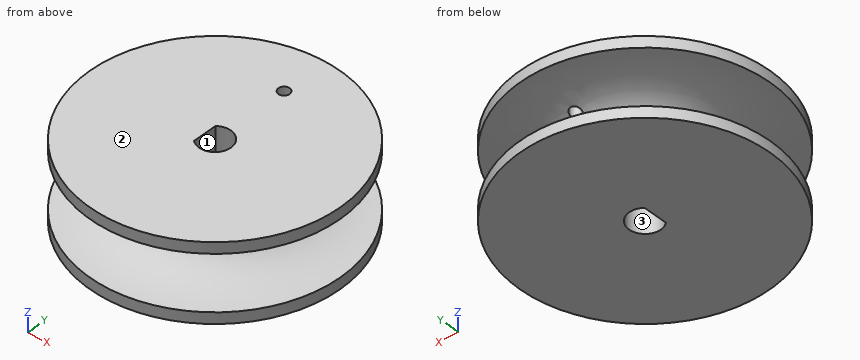
```python
from build123d import *

# Parameters (mm, degrees)
BOSS_EXTRUDE1_START = -7
BOSS_EXTRUDE1_DEPTH = 7
SKETCH8_R           = 0.5
CUT_EXTRUDE1_DEPTH  = 3


with BuildPart() as part:
    # Sketch4 → Revolve1 (revolve)
    with BuildSketch(Plane(origin=(0, 0, 0), x_dir=(0, 0, -1), z_dir=(1, 0, 0)), mode=Mode.PRIVATE) as revolve1_sk:
        with BuildLine():
            Line((-2.5, 11.25), (-3.5, 11.25))
            Line((-3.5, 11.25), (-3.5, 1.425))
            Line((-3.5, 1.425), (3.5, 1.425))
            Line((3.5, 1.425), (3.5, 11.25))
            Line((3.5, 11.25), (2.5, 11.25))
            add(Edge.make_bspline(
                [(0, 5.689829973), (2.5, 5.689829973), (2.5, 11.25)],
                knots=[0, 0, 0, 1.570796327, 1.570796327, 1.570796327], degree=2, weights=[1, 0.707106781, 1]))
            add(Edge.make_bspline(
                [(-2.5, 11.25), (-2.5, 5.689829973), (0, 5.689829973)],
                knots=[4.71238898, 4.71238898, 4.71238898, 6.283185307, 6.283185307, 6.283185307], degree=2, weights=[1, 0.707106781, 1]))
        make_face()
    revolve(revolve1_sk.sketch.rotate(Axis((0, 0, 0), (0, 0, -1)), 90), axis=Axis((0, 0, 0), (0, 0, -1)))

    # Sketch7 → Boss-Extrude1 (add)
    with BuildSketch(Plane.XY.offset(3.5).offset(BOSS_EXTRUDE1_START)):
        with BuildLine():
            Line((-0.925, 1.083974169), (-0.925, -1.083974169))
            ThreePointArc((-0.925, -1.083974169), (-1.425, 0), (-0.925, 1.083974169))
        make_face()
    extrude(amount=BOSS_EXTRUDE1_DEPTH)

    # Sketch8 → Cut-Extrude1 (cut)
    with BuildSketch(Plane.XY.offset(3.5)):
        with Locations((0, 7)):
            Circle(SKETCH8_R)
    extrude(amount=-CUT_EXTRUDE1_DEPTH, mode=Mode.SUBTRACT)


solid = part.part
```
For this review, take the finished solid that the model builds, in its own axes (mm). Face numbers are marked on the shaded views. Round coordinates to 2 decimals unless told otherwise and drop trailing zeros. Write each question's results on one line, items separated by ' | '.
Item 1: Take a section at A-A on x = 0. Count the separate pieces of the cut face and the enclosed holes in it, then the cut area to 3 significant figures.
Calculated:
separate pieces: 3 | enclosed holes: 0 | area: 92.0 mm^2
Item 2: Draft analysis for pull direction Y (two halves, no side actions). For the marked faces 1, 2 and 3, state which applies: pulls with the +Y half, pulls with the -Y half, needs draft (parallel to the pull), parting line crosses it, or undercut.
Calculated:
face 1: undercut | face 2: needs draft | face 3: undercut
Item 3: To check wall thickness, follow line 1 along Z through (x, y) = (-9, -6.25); line 2 along X through (y, z) = (0.5, 0.25) (3 decimals); line 3 along Z through (x, y) = (-8.25, 2.5). State the ranges of each line that lie inside material, in increasing order. Write a range as from..to.
Calculated:
line 1: z = -3.5..-2.5, 2.5..3.5 | line 2: x = -5.696..-0.925, 1.334..5.696 | line 3: z = -3.5..-2.2, 2.2..3.5
Item 4: For pin 1 (1.7 mm diameter, centred on y = 0.5, z = -0.5, fed in from +X); pin 2 (4 mm diameter, centred on x = -7, z = -1.5, fed in from +Y); pin 3 (1.5 mm diameter, centred on x = 3, z = 2, fed in from +Y), all flat-tipped, find the tip position at first contact; note any pin that passes through.
Calculated:
pin 1: stops at x = 6.55 | pin 2: stops at y = 9.94 | pin 3: stops at y = 10.98
